Check sheet for the drawn part. Datum: minimum x, y, z corner. Units: mm. A direction names the side the tool comes from. Round coordinates to 2 decimals unless told otherwise and drop trailing zeros. Order: outer loops, then holes, each group sorted by start corner. A loop starts at its lowest first (then second) coordinate and runs counter-clockwise, first axis right, second up. Notation, with made-up numbers: (49.5, -30) - (89.5, -30) arc R23 cw to (89.5, 3) - close; hole circle Ø5 at (15, 15.5). An arc over 180 degrees is marked (long way). Write each question's results on one line, items separated by ' | '.
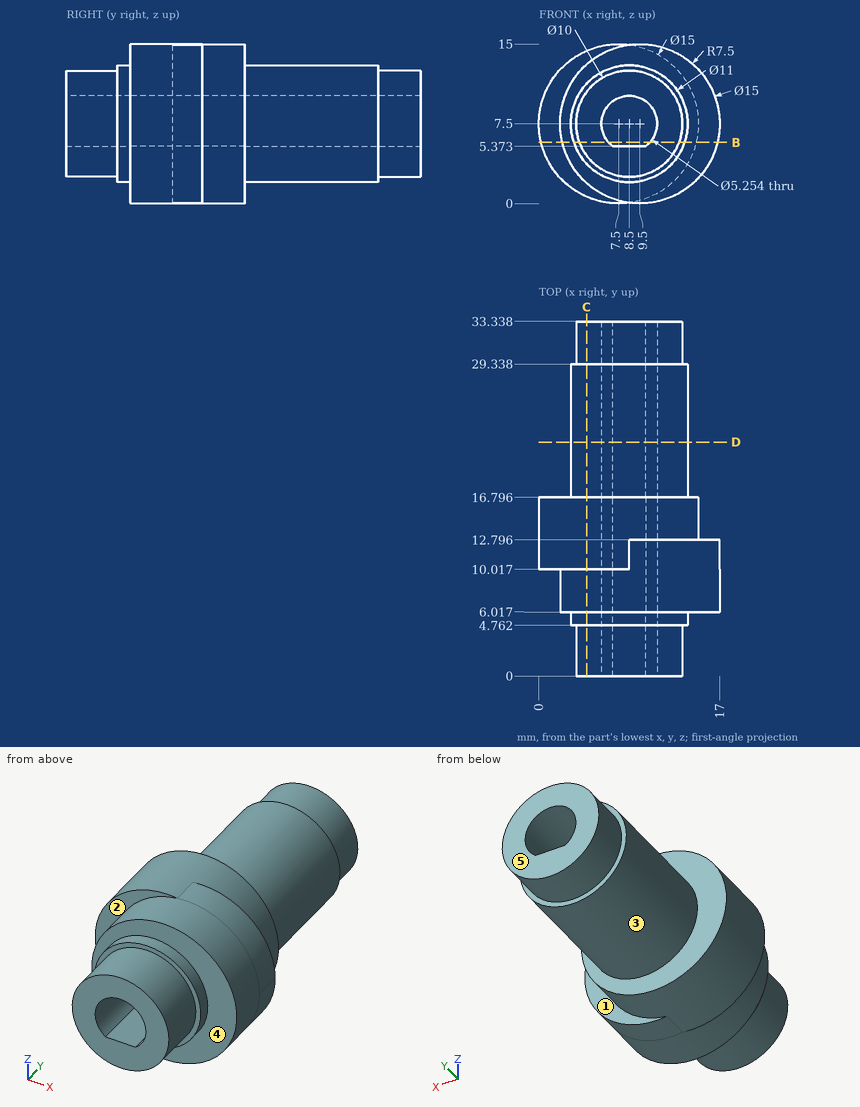
(1) Access from +Z, -Z, +X, -X, +Y, -Y to the whole of each face (thin tool, end or side, straight path). Record for the marked faces 1, 2, 3, 4 and 5.
Answers follow:
face 1: +X, +Y | face 2: -X, -Y | face 3: +Y | face 4: -Y | face 5: +Z, -Z, +X, -X, +Y
(2) Depth check by flat-ended pin: pin 1 Ø1.5 at (x, z) = (13, 3) entering from -Y; pin 2 Ø8 at (y, z) = (29.5, 8.5) entering from -X; pin 3 Ø1 at (y, z) = (8.5, 9) entering from -X; pin 4 Ø8 at (x, z) = (11.5, 8.5) entering from -Y. Enter the tip coordinate at first touch or a pass-through.
Answers follow:
pin 1: y = 6.02 | pin 2: x = 3 | pin 3: x = 2.07 | pin 4: y = 0
(3) Section check D-D (y = 22). Record the cut outline in (x, z) (1 decimal).
Answers follow:
outline: circle Ø11 at (8.5, 7.5); hole (7, 5.4) - (10, 5.4) arc R2.6 ccw (long way) to start
(4) Section check B-B (z = 5.75). Record the cut outline in (x, y) (1 decimal), then the cut area to 3 significant figures.
Answers follow:
outline: (0.2, 10) - (2.2, 10) - (2.2, 6) - (3.3, 6) - (3.3, 4.8) - (3.8, 4.8) - (3.8, 0) - (6.5, 0) - (6.5, 33.3) - (3.8, 33.3) - (3.8, 29.3) - (3.3, 29.3) - (3.3, 16.8) - (0.2, 16.8) - close; (10.5, 0) - (13.2, 0) - (13.2, 4.8) - (13.7, 4.8) - (13.7, 6) - (16.8, 6) - (16.8, 12.8) - (14.8, 12.8) - (14.8, 16.8) - (13.7, 16.8) - (13.7, 29.3) - (13.2, 29.3) - (13.2, 33.3) - (10.5, 33.3) - close | area: 258 mm²
(5) Material ranges on line 1 (X direction, y = 3.25, z = 7.5); line 2 (X direction, y = 23.5, z = 7.5); line 3 (Y direction, x = 13.5, z = 1.5) (1 decimal), recorded low to high.
Answers follow:
line 1: 3.5 to 5.87, 11.13 to 13.5 | line 2: 3 to 5.87, 11.13 to 14 | line 3: 6 to 12.8
(6) Section check C-C (x = 4.5). Record the cut outline in (y, z) (1 decimal).
Answers follow:
outline: (0, 4.5) - (4.8, 4.5) - (4.8, 3.7) - (6, 3.7) - (6, 1.9) - (10, 1.9) - (10, 0.6) - (16.8, 0.6) - (16.8, 3.7) - (29.3, 3.7) - (29.3, 4.5) - (33.3, 4.5) - (33.3, 10.5) - (29.3, 10.5) - (29.3, 11.3) - (16.8, 11.3) - (16.8, 14.4) - (10, 14.4) - (10, 13.1) - (6, 13.1) - (6, 11.3) - (4.8, 11.3) - (4.8, 10.5) - (0, 10.5) - close
